Autodesk Fusion 360 part; units mm, degrees
sketch "3D-printed conduit outline" plane through (0, 0, 0) normal (0, 1, 0) x (1, 0, 0)
  line L0 (0, 0) -> (16, 0)
  line L1 (16, 0) -> (16, -14)
  line L2 (16, -14) -> (0, -14)
  line L3 (0, -14) -> (0, 0)
  line L4 (2, -14) -> (14, -14)
  line L5 (14, -14) -> (14, -2)
  line L6 (14, -2) -> (2, -2)
  line L7 (2, -2) -> (2, -14)
  dimension "d8" = 14
  dimension "d9" = 16
  dimension "d10" = 2
  dimension "d11" = 2
  dimension "d12" = 2
extrude "Extrude1" add sketch "3D-printed conduit outline" along normal blind 161.69 contours L0 L1 L2 L3 L5 L6 L7
sketch "Magnet holders" plane through (0, 0, 14) normal (0, 0, 1) x (-1, 0, 0)
  line L0 (0, 0) -> (-2, 0)
  line L1 (-2, 0) -> (-2, -161.69)
  line L2 (-2, -161.69) -> (0, -161.69)
  line L3 (0, -161.69) -> (0, 0)
  line L4 (-14, 0) -> (-16, 0)
  line L5 (-16, 0) -> (-16, -161.69)
  line L6 (-16, -161.69) -> (-14, -161.69)
  line L7 (-14, -161.69) -> (-14, 0)
  circle A0 centre (-2.5, -2.5) radius 2.5
  circle A1 centre (-2.5, -2.5) radius 1.75
  line L8 (-14, 0) -> (-2, 0)
  line L9 (0, 0) -> (-2.5, 0)
  line L10 (-2.5, 0) -> (-2.5, -5)
  line L11 (-2.5, -5) -> (0, -5)
  line L12 (0, -5) -> (0, 0)
  circle A2 centre (-13.5, -2.5) radius 2.5
  circle A3 centre (-13.5, -2.5) radius 1.75
  line L13 (-16, 0) -> (-13.5, 0)
  line L14 (-13.5, 0) -> (-13.5, -5)
  line L15 (-13.5, -5) -> (-16, -5)
  line L16 (-16, -5) -> (-16, 0)
  circle A4 centre (-2.5, -54.73) radius 1.75
  circle A5 centre (-2.5, -54.73) radius 2.5
  line L17 (-2.5, -52.23) -> (-2.5, -57.23)
  line L18 (-2.5, -57.23) -> (0, -57.23)
  line L19 (0, -57.23) -> (0, -52.23)
  line L20 (0, -52.23) -> (-2.5, -52.23)
  circle A6 centre (-13.5, -54.73) radius 1.75
  circle A7 centre (-13.5, -54.73) radius 2.5
  line L21 (-13.5, -52.23) -> (-13.5, -57.23)
  line L22 (-13.5, -57.23) -> (-16, -57.23)
  line L23 (-16, -57.23) -> (-16, -52.23)
  line L24 (-16, -52.23) -> (-13.5, -52.23)
  circle A8 centre (-2.5, -106.96) radius 1.75
  circle A9 centre (-2.5, -106.96) radius 2.5
  line L25 (-2.5, -104.46) -> (-2.5, -109.46)
  line L26 (-2.5, -109.46) -> (0, -109.46)
  line L27 (0, -109.46) -> (0, -104.46)
  line L28 (0, -104.46) -> (-2.5, -104.46)
  circle A10 centre (-13.5, -106.96) radius 1.75
  circle A11 centre (-13.5, -106.96) radius 2.5
  line L29 (-13.5, -104.46) -> (-13.5, -109.46)
  line L30 (-13.5, -109.46) -> (-16, -109.46)
  line L31 (-16, -109.46) -> (-16, -104.46)
  line L32 (-16, -104.46) -> (-13.5, -104.46)
  circle A12 centre (-2.5, -159.19) radius 1.75
  circle A13 centre (-2.5, -159.19) radius 2.5
  line L33 (-2.5, -156.69) -> (-2.5, -161.69)
  line L34 (-2.5, -161.69) -> (0, -161.69)
  line L35 (0, -161.69) -> (0, -156.69)
  line L36 (0, -156.69) -> (-2.5, -156.69)
  circle A14 centre (-13.5, -159.19) radius 1.75
  circle A15 centre (-13.5, -159.19) radius 2.5
  line L37 (-13.5, -156.69) -> (-13.5, -161.69)
  line L38 (-13.5, -161.69) -> (-16, -161.69)
  line L39 (-16, -161.69) -> (-16, -156.69)
  line L40 (-16, -156.69) -> (-13.5, -156.69)
  dimension "d15" = 5
  dimension "d16" = 3.5
  dimension "d17" = 5
  dimension "d18" = 3.5
  dimension "d21" = 0
  dimension "d22" = -156.69
extrude "Extrude2" add sketch "Magnet holders" against normal blind 3 contours A2 A3 L14 | L7 A2 A3 L14 | L7 L8 A2 L13 | L1 A0 L8 L9 | L1 A0 A1 L10 | A0 A1 L10 | L1 A0 A1 L10 | L1 A0 L11 | L1 A1 L10 | A1 L10 | L7 A3 L14 | A3 L14 | L1 A5 L20 | L7 A2 L15 | L7 A2 A3 L14 | L1 A4 A5 L17 | L1 A4 A5 L17 | L1 A5 L18 | A4 A5 L17 | L1 A4 L17 | A4 L17 | L7 A7 L24 | L1 A9 L28 | L7 A6 A7 L21 | A6 A7 L21 | L1 A8 A9 L25 | L1 A8 A9 L25 | L1 A9 L26 | A8 A9 L25 | L7 A6 L21 | A6 L21 | L7 A7 L22 | L7 A6 A7 L21 | L1 A8 L25 | A8 L25 | L1 A13 L36 | L7 A11 L32 | L1 A12 A13 L33 | L1 A12 A13 L33 | L1 A13 L34 | A12 A13 L33 | L7 A10 A11 L29 | L7 A11 L30 | L7 A10 A11 L29 | A10 A11 L29 | L1 A12 L33 | A12 L33 | L7 A10 L29 | A10 L29 | L7 A15 L40 | L7 A14 A15 L37 | L7 A15 L38 | L7 A14 A15 L37 | A14 A15 L37 | L7 A14 L37 | A14 L37
extrude "Extrude3" cut sketch "Magnet holders" against normal blind 1 contours L1 A1 | L1 A1 L10 | A1 L10 | L7 A3 L14 | A3 L14 | L7 A3 | L1 A4 | L1 A4 L17 | A4 L17 | L7 A6 L21 | L7 A6 | A6 L21 | L1 A8 | L1 A8 L25 | A8 L25 | L1 A12 | L1 A12 L33 | A12 L33 | L7 A10 L29 | L7 A10 | A10 L29 | L7 A14 L37 | L7 A14 | A14 L37
chamfer "Chamfer1" distance 1 angle 45 2 edges at (2, 80.845, 2) (14, 80.845, 2)
chamfer "Chamfer2" distance 2.9999 angle 45 8 edges at (2, 2.5, 11) (2, 54.73, 11) (2, 106.96, 11) (2, 159.19, 11) (14, 2.5, 11) (14, 54.73, 11) (14, 106.96, 11) (14, 159.19, 11)
equation "conduit_length = 161.69 mm"
equation "conduit_width = 16 mm"
equation "conduit_height = 16 mm"
equation "conduit_wall_thickness = 2 mm"
equation "magnet_diameter = 3 mm"
equation "magnet_height = 1 mm"
equation "d8 = conduit_height - conduit_wall_thickness"
equation "d9 = conduit_width"
equation "d10 = conduit_wall_thickness"
equation "d11 = conduit_wall_thickness"
equation "d12 = conduit_wall_thickness"
equation "d13 = conduit_length"
equation "d15 = magnet_diameter + 2 mm"
equation "d16 = magnet_diameter + 0.5 mm"
equation "d17 = magnet_diameter + 2 mm"
equation "d18 = magnet_diameter + 0.5 mm"
equation "d22 = -conduit_length + ( magnet_diameter + 2 mm )"
equation "d23 = -( magnet_height + 2 mm )"
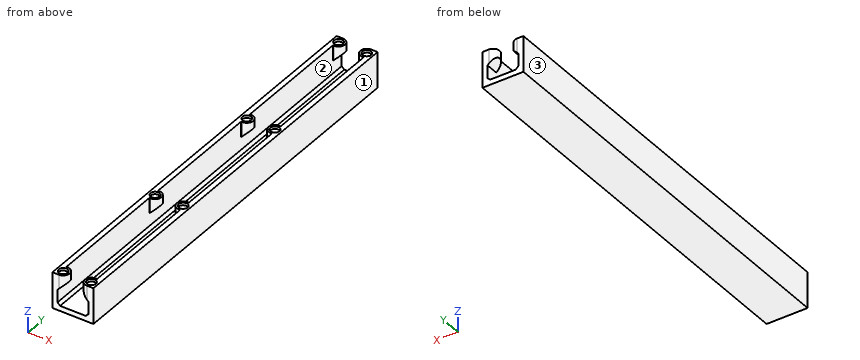
Geometry check sheet. Reference: the model listing, model coordinates, mm. Face numbers are marked on the shaded views. Give positions to 0.01 mm unless a question says otherwise; leave off trailing zeros. Write each loop counter-clockwise with the first axis right and the second up, starting at its lowest first coordinate (ties: lowest second). Pieces come first, ordered by that corner, then holes.
1) Section check A-A, the plane y = 65.5. Record the boundary of the cut face in (x, z), and give its area (3 significant figures).
2) Release check for a two-part mould opening along X. For the marked faces 1, 2 and 3 record: pulls with the +X half, pulls with the -X half, needs draft (parallel to the pull), parting line crosses it, or undercut.
3) Gauge pin test, flat ends, axial feed: pin 1 (5 mm diameter, centred on x = 9, y = 71.5, fed in from +Z); pin 2 (3 mm diameter, centred on x = 2.5, y = 54.73, fed in from +Z). Record the tip position at first contact, or that the pin passes through.
4) Material ranges on L1, parallel to X at y = 106.96, z = 13.85; L2, parallel to Y at x = 13.75, z = 9.25; L3, parallel to X at y = 35, z = 6, recorded low to high.
Computed:
1. outline: (0, 0) - (16, 0) - (16, 14) - (14, 14) - (14, 3) - (13, 2) - (3, 2) - (2, 3) - (2, 14) - (0, 14) - close
1. area: 81.0 mm2
2. face 1: pulls with the +X half
2. face 2: undercut
2. face 3: pulls with the -X half
3. pin 1: stops at z = 2
3. pin 2: stops at z = 13
4. L1: x = 0 to 0.75, 4.25 to 5, 11 to 11.75, 15.25 to 16
4. L2: y = 0 to 5, 52.23 to 57.23, 104.46 to 109.46, 156.69 to 161.69
4. L3: x = 0 to 2, 14 to 16
